Design review of the part built by this model. Coordinates are the model's own, in mm. A direction names the side the tool comes from. Round coordinates to 2 decimals unless told otherwise and drop trailing zeros. Loops run counter-clockwise (first coordinate to the right, second up) from the corner with the lowest first, then second, coordinate; pieces in that order, holes last. Notation, with made-up numbers: M 71,-39 L 87,-39 A20 ccw 87,-18 Z; hole C -39,11 d7. An arc over 180 degrees is marked long. Use a Markdown table: item, result.
Autodesk Inventor part; units mm, degrees
ref_plane "YZ Plane" through (0, 0, 0) normal (1, 0, 0) x (0, 1, 0)
ref_plane "XZ Plane" through (0, 0, 0) normal (0, 1, 0) x (-1, 0, 0)
ref_plane "XY Plane" through (0, 0, 0) normal (0, 0, 1) x (1, 0, 0)
sketch "草图1" plane through (0, 0, 0) normal (0, 1, 0) x (-1, 0, 0)
  line L0 (110.5, 55.5) -> (-110.5, 55.5)
  line L1 (-110.5, 55.5) -> (-110.5, -55.5)
  line L2 (-110.5, -55.5) -> (110.5, -55.5)
  line L3 (110.5, -55.5) -> (110.5, 55.5)
  line L4 (0, 7.5575) -> (0, -11)
  line L5 (8.5019, 0) -> (-7, 0)
  point P0 (0, 0)
  point P1 (0, 0)
  point P2 (0, 0)
  dimension "d0" = 221
  dimension "d1" = 111
extrude "拉伸1" add sketch "草图1" along normal blind 6
fillet "圆角1" radius 10.1 1 edges at (-110.5, 3, -55.5)
sketch "草图2" plane through (0, 6, 0) normal (0, 1, 0) x (1, 0, 0)
  circle A0 centre (-64.5, 9.5) radius 10.05
  line L0 (110.5, 55.5) -> (-100.4, 55.5)
  line L1 (-110.5, 45.4) -> (-110.5, -55.5)
  point P0 (0, 0)
  dimension "d5" = 20.1
  dimension "d6" = 46
  dimension "d7" = 46
extrude "拉伸2" cut sketch "草图2" against normal blind 6
sketch "草图3" plane through (0, 6, 0) normal (0, 1, 0) x (1, 0, 0)
  line L0 (100.5, 55.5) -> (120.5, 55.5)
  line L1 (120.5, 55.5) -> (120.5, -55.5)
  line L2 (120.5, -55.5) -> (100.5, -55.5)
  line L3 (100.5, -55.5) -> (100.5, 55.5)
  line L4 (110.5, -55.5) -> (110.5, 55.5)
  circle A0 centre (116.5, 25.5) radius 2.1
  circle A1 centre (116.5, -25.5) radius 2.1
  point P0 (0, 0)
  dimension "d10" = 20
  dimension "d11" = 10
  dimension "d12" = 4.2
  dimension "d13" = 4.2
  dimension "d14" = 4
  dimension "d15" = 4
  dimension "d16" = 30
  dimension "d17" = 30
extrude "拉伸3" add sketch "草图3" along normal blind 6
fillet "圆角2" radius 6 1 edges at (100.5, 6, 0)
sketch "草图4" plane through (0, 0, 0) normal (0, -1, 0) x (1, 0, 0)
  circle A0 centre (-50.5, 40.5) radius 2.1
  circle A1 centre (49.5, 40.5) radius 2.1
  line L0 (-110.5, 55.5) -> (110.5, 55.5)
  line L1 (-110.5, -45.4) -> (-110.5, 55.5)
  point P0 (0, 0)
  dimension "d21" = 4.2
  dimension "d22" = 4.2
  dimension "d23" = 15
  dimension "d24" = 15
  dimension "d25" = 60
  dimension "d26" = 100
extrude "拉伸4" cut sketch "草图4" against normal blind 6
sketch "草图5" plane through (0, 0, 0) normal (0, -1, 0) x (1, 0, 0)
  circle A0 centre (-50.5, 40.5) radius 2.1
  circle A1 centre (-50.5, 40.5) radius 3.6
  circle A2 centre (49.5, 40.5) radius 2.1
  circle A3 centre (49.5, 40.5) radius 3.6
  point P0 (0, 0)
  dimension "d29" = 7.2
  dimension "d30" = 7.2
extrude "拉伸5" cut sketch "草图5" against normal blind 4 contours A0 | A1 | A2 | A3
properties part number "底板_C"
1. The part is to be moulded in two halves that separate along Z. For faces 1 (the face through (-107.46, 3.04, -52.62)), 2 (the face through (-7, 6, 1)), 3 (the face through (118.503, 8.958, 26.131)), say which applies: pulls with the +Z half, pulls with the -Z half, needs draft (parallel to the pull), parting line crosses it, or undercut.
Check values:
| item | result |
|---|---|
| face 1 | pulls with the -Z half |
| face 2 | needs draft |
| face 3 | undercut |
2. Insertion check: pin 1 (2.5 mm diameter, centred on x = 49.5, z = 40.5, fed in from -Y); pin 2 (5 mm diameter, centred on y = 2.5, z = 28.5, fed in from +X); pin 3 (8 mm diameter, centred on x = 118, z = -19, fed in from -Y); pin 4 (6.5 mm diameter, centred on x = -50.5, z = 40.5, fed in from -Y). Each pin has a flat end and moves straight along its axis. Give the tip position at first contact, or say it passes through.
Check values:
| item | result |
|---|---|
| pin 1 | passes through |
| pin 2 | stops at x = 110.5 |
| pin 3 | stops at y = 6 |
| pin 4 | stops at y = 4 |
3. Wall thickness on line 1 along Z through (x, y) = (-50.5, 1.7); line 2 along Y through (x, z) = (-14, -22.5); line 3 along X through (y, z) = (5, -30): over which ranges is each line inside the solid? List them lowest first. Write a range as from..to.
Check values:
| item | result |
|---|---|
| line 1 | z = -55.5..36.9, 44.1..55.5 |
| line 2 | y = 0..6 |
| line 3 | x = -110.5..110.5 |
4. Take a section at C-C on x = 116.5. Give the boundary of the cut face in (y, z), and give its area (3 significant figures).
Check values:
| item | result |
|---|---|
| outline | M 6,-55.5 L 12,-55.5 L 12,-27.6 L 6,-27.6 Z; M 6,-23.4 L 12,-23.4 L 12,23.4 L 6,23.4 Z; M 6,27.6 L 12,27.6 L 12,55.5 L 6,55.5 Z |
| area | 616 mm² |
5. Take a section at B-B on z = 40.5. Count the separate pieces of the cut face and the enclosed holes in it, and give its area (3 significant figures).
Check values:
| item | result |
|---|---|
| separate pieces | 3 |
| enclosed holes | 0 |
| area | 1,380 mm² |
6. Machinability: for faces 4 (the face through (115, 6, -1)), 5 (the face through (3, 3, 55.5)), 6 (the face through (52, 4, 41)), which of the approach directions +Z, -Z, +X, -X, +Y, -Y give a long, thin tool a straight path to every point of the face, cutting with its end or side? Answer none if there is none.
Check values:
| item | result |
|---|---|
| face 4 | +Z, -Z, +X, -Y |
| face 5 | +Z, +X, -X, +Y, -Y |
| face 6 | -Y |
7. Take a section at A-A on x = 49.5. Give the boundary of the cut face in (y, z), and give its area (3 significant figures).
Check values:
| item | result |
|---|---|
| outline | M 0,-55.5 L 6,-55.5 L 6,38.4 L 4,38.4 L 4,36.9 L 0,36.9 Z; M 0,44.1 L 4,44.1 L 4,42.6 L 6,42.6 L 6,55.5 L 0,55.5 Z |
| area | 629 mm² |
